Input: part model. Units: mm. Frame: model coordinates. A direction names the side the tool comes from. Give positions to 0.01 mm unless a question says otherwise; leave off trailing zeros. Order: outer loops, then holes, each group sorted by start corner. A loop starts at its lowest first (then second) coordinate and runs counter-clockwise, first axis right, second up.
```python
from build123d import *

# Parameters (mm, degrees)
SKETCH1_W               = 176
SKETCH1_H               = 81
BOSS_EXTRUDE1_DEPTH     = 3
FILLET1_R               = 5
SKETCH2_W               = 170
SKETCH2_H               = 70
BOSS_EXTRUDE2_DEPTH     = 6
SKETCH3_R               = 1.6
CUT_EXTRUDE1_DEPTH      = 98.057972367
SKETCH5_R               = 3
CUT_EXTRUDE5_DEPTH      = 2
MIRROR2_COPY_1_SKETCH_R = 1.6
MIRROR2_COPY_1_DEPTH    = 98.057972367
MIRROR2_COPY_2_SKETCH_R = 3
MIRROR2_COPY_2_DEPTH    = 2


with BuildPart() as part:
    # Sketch1 → Boss-Extrude1 (new body)
    with BuildSketch(Plane(origin=(0, 0, 0), x_dir=(1, 0, 0), z_dir=(0, 1, 0))):
        Rectangle(SKETCH1_W, SKETCH1_H)
    extrude(amount=BOSS_EXTRUDE1_DEPTH)

    # Fillet1
    fillet1_edges = [part.edges().sort_by_distance(p)[0] for p in [
        (-88, 1.5, -40.5),
        (-88, 1.5, 40.5),
        (88, 1.5, 40.5),
        (88, 1.5, -40.5),
    ]]
    fillet(fillet1_edges, radius=FILLET1_R)

    # Sketch2 → Boss-Extrude2 (add)
    with BuildSketch(Plane.XZ):
        Rectangle(SKETCH2_W, SKETCH2_H)
    extrude(amount=-BOSS_EXTRUDE2_DEPTH)

    # Sketch3 → Cut-Extrude1 (cut, through all)
    with BuildSketch(Plane(origin=(0, 6, 0), x_dir=(1, 0, 0), z_dir=(0, 1, 0))):
        with Locations(Location((-80, 31, 0), (0, 0, 270))):
            Circle(SKETCH3_R)
    cut_extrude1 = extrude(amount=-CUT_EXTRUDE1_DEPTH, mode=Mode.SUBTRACT)

    # Sketch5 → Cut-Extrude5 (cut)
    with BuildSketch(Plane.XZ):
        with Locations(Location((-80, -31, 0), (0, 0, 270))):
            Circle(SKETCH5_R)
    cut_extrude5 = extrude(amount=-CUT_EXTRUDE5_DEPTH, mode=Mode.SUBTRACT)

    # Mirror1: Cut-Extrude1, Cut-Extrude5 across plane
    add(cut_extrude1.mirror(Plane.XY), mode=Mode.SUBTRACT)
    add(cut_extrude5.mirror(Plane.XY), mode=Mode.SUBTRACT)

    # Mirror2: Cut-Extrude1, Cut-Extrude5 across plane
    add(cut_extrude1.mirror(Plane(origin=(0, 0, 0), x_dir=(0, 0, 1), z_dir=(1, 0, 0))), mode=Mode.SUBTRACT)
    add(cut_extrude5.mirror(Plane(origin=(0, 0, 0), x_dir=(0, 0, 1), z_dir=(1, 0, 0))), mode=Mode.SUBTRACT)

    # Mirror2 copy 1 sketch → Mirror2 copy 1 (cut, through all)
    with BuildSketch(Plane(origin=(0, 6, 0), x_dir=(-1, 0, 0), z_dir=(0, 1, 0))):
        with Locations(Location((-80, 31, 0), (0, 0, 270))):
            Circle(MIRROR2_COPY_1_SKETCH_R)
    extrude(amount=-MIRROR2_COPY_1_DEPTH, mode=Mode.SUBTRACT)

    # Mirror2 copy 2 sketch → Mirror2 copy 2 (cut)
    with BuildSketch(Plane(origin=(0, 0, 0), x_dir=(-1, 0, 0), z_dir=(0, -1, 0))):
        with Locations(Location((-80, -31, 0), (0, 0, 270))):
            Circle(MIRROR2_COPY_2_SKETCH_R)
    extrude(amount=-MIRROR2_COPY_2_DEPTH, mode=Mode.SUBTRACT)


solid = part.part
```
1) Cut plane C-C (y = 4.3). Return the cut outline in (x, z), then the cut area to 3 significant figures.
2) Cut plane A-A (x = 80). Return the cut outline in (y, z), then the cut area to 3 significant figures.
3) Cut plane B-B (z = -31). Return the cut outline in (x, y), then the cut area to 3 significant figures.
4) Pull-direction query (Z, two-part tool) for faces 3 (the face through (-81.3, 2, 32.3)), 4 (the face through (-85, 4, 0)), 5 (the face through (-1, 4, -35)); classes: pulls with the +Z half, pulls with the -Z half, needs draft (parallel to the pull), parting line crosses it, or undercut.
5) First-contact query: P1, Ø5, axis at x = 80, z = -31, coming from the -Y side; P2, Ø0.9, axis at y = 5, z = -4, coming from the -X side; P3, Ø2.5, axis at x = 9.5, y = 5, coming from the -Z side. Flat tips, straight axial feed; report the tip coordinate or a pass-through.
6) Reachability of faces 1 (the face through (-1, 6, 0)), 2 (the face through (81.3, 2, 32.3)) from +Z, -Z, +X, -X, +Y, -Y: full face, straight path, thin tool, end or side. Return the list, or none.
7) Line query: probe 1 along X at (y, z) = (0.8, 31); probe 2 along Z at (x, y) = (80, 0.45); probe 3 along Z at (x, y) = (80, 2.9). Output: solid intervals per line, ascending.
8) Cut plane D-D (x = -70). Return the cut outline in (y, z), then the cut area to 3 significant figures.
Geometry says:
1. outline: (-85, -35) - (85, -35) - (85, 35) - (-85, 35) - close; hole circle Ø3.2 at (-80, -31); hole circle Ø3.2 at (-80, 31); hole circle Ø3.2 at (80, -31); hole circle Ø3.2 at (80, 31)
1. area: 11,900 mm2
2. outline: (0, -40.5) - (3, -40.5) - (3, -35) - (6, -35) - (6, -32.6) - (2, -32.6) - (2, -34) - (0, -34) - close; (0, -28) - (2, -28) - (2, -29.4) - (6, -29.4) - (6, 29.4) - (2, 29.4) - (2, 28) - (0, 28) - close; (0, 34) - (2, 34) - (2, 32.6) - (6, 32.6) - (6, 35) - (3, 35) - (3, 40.5) - (0, 40.5) - close
2. area: 403 mm2
3. outline: (-88, 0) - (-83, 0) - (-83, 2) - (-81.6, 2) - (-81.6, 6) - (-85, 6) - (-85, 3) - (-88, 3) - close; (-78.4, 2) - (-77, 2) - (-77, 0) - (77, 0) - (77, 2) - (78.4, 2) - (78.4, 6) - (-78.4, 6) - close; (81.6, 2) - (83, 2) - (83, 0) - (88, 0) - (88, 3) - (85, 3) - (85, 6) - (81.6, 6) - close
3. area: 988 mm2
4. face 3: undercut
4. face 4: needs draft
4. face 5: pulls with the -Z half
5. P1: stops at y = 2
5. P2: stops at x = -85
5. P3: stops at z = -35
6. face 1: +Z, -Z, +X, -X, +Y
6. face 2: -Y
7. probe 1: x = -88 to -83, -77 to 77, 83 to 88
7. probe 2: z = -40.5 to -34, -28 to 28, 34 to 40.5
7. probe 3: z = -40.5 to -32.6, -29.4 to 29.4, 32.6 to 40.5
8. outline: (0, -40.5) - (3, -40.5) - (3, -35) - (6, -35) - (6, 35) - (3, 35) - (3, 40.5) - (0, 40.5) - close
8. area: 453 mm2
